Input: dimensioned drawing with shaded views. Units: mm. Origin: part minimum x, y, z. A direction names the side the tool comes from. Coordinates: 2 decimals unless noted, no trailing zeros. Loops run counter-clockwise (first coordinate to the right, second up) from the corner with the lowest first, then second, coordinate; pieces in that order, holes last.
Item 1: Pull-direction query (Y, two-part tool) for the marked faces 1, 2 and 3; classes: released by +Y, released by -Y, zero draft, split by the parting line, or undercut.
Item 2: Ray query, line 1 along Z through (x, y) = (4.5, 23.5); line 2 along X through (y, z) = (40, 30); line 3 along Y through (x, z) = (16, 15.5). Return the intervals inside material, ascending.
Item 3: Contact query for flat-ended pins moving along their axis: P1, Ø3, axis at x = 33.5, z = 28.5, coming from the +Y side; P2, Ø1.5, axis at x = 42.5, y = 14.5, coming from the +Z side; P3, Ø6, axis at x = 38, z = 25.5, coming from the +Y side (1 decimal). Output: stop coordinate, or through.
Item 4: Section C-C on x = 45. Return loops of the section in (y, z) (1 decimal).
Item 5: Section B-B on x = 32. Return loops of the section in (y, z) (1 decimal), and give its area (3 significant figures).
Item 6: Section A-A on x = 17. Return loops of the section in (y, z), and give its area (3 significant figures).
Item 7: Reachability of the marked faces 4, 5 and 6 from +Z, -Z, +X, -X, +Y, -Y: full face, straight path, thin tool, end or side. Return the list, or none.
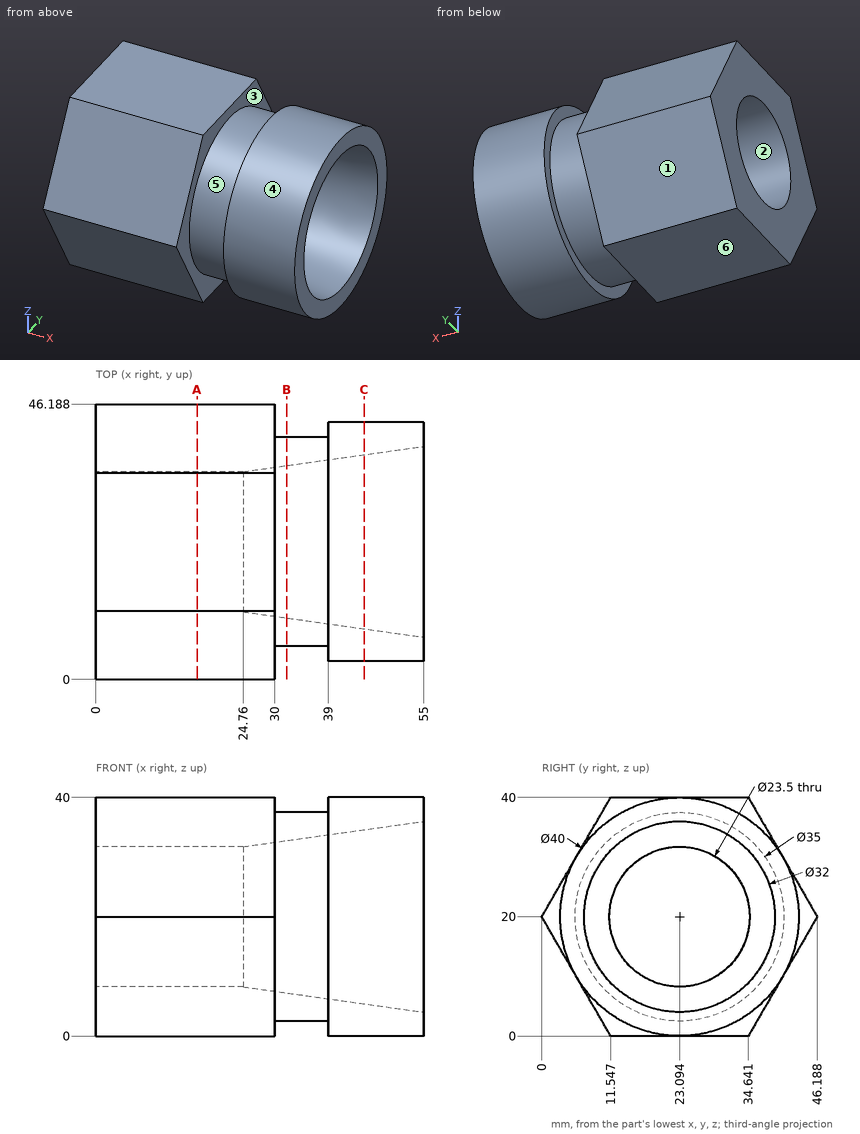
Results found:
1. face 1: released by +Y
1. face 2: undercut
1. face 3: zero draft
2. line 1: z = 0 to 8.26, 31.74 to 40
2. line 2: x = 0 to 30, 39 to 55
2. line 3: y = 2.6 to 12.24, 33.95 to 43.59
3. P1: stops at y = 39.13
3. P2: stops at z = 38.4
3. P3: stops at y = 42.9
4. outline: circle Ø40 at (23.1, 20); hole circle Ø29.2 at (23.1, 20)
5. outline: circle Ø35 at (23.1, 20); hole circle Ø25.5 at (23.1, 20)
5. area: 450 mm2
6. outline: (0, 20) - (11.55, 0) - (34.64, 0) - (46.19, 20) - (34.64, 40) - (11.55, 40) - close; hole circle Ø23.5 at (23.09, 20)
6. area: 952 mm2
7. face 4: +X
7. face 5: none
7. face 6: -Z, +X, -X, +Y, -Y
